```python
from build123d import *

# Parameters (mm, degrees)
CYLINDER_R        = 1.5
CYLINDER_DEPTH    = 8
CYLINDER002_R     = 1
CYLINDER002_DEPTH = 7
BOX005_W          = 11
BOX005_H          = 10
BOX005_DEPTH      = 6
FILLET001_R       = 3
BOX_W             = 14
BOX_H             = 30
BOX_DEPTH         = 24
BOX003_W          = 11
BOX003_H          = 3
BOX003_DEPTH      = 11
BOX004_W          = 11
BOX004_H          = 9
BOX004_DEPTH      = 7
CYLINDER001_R     = 1
CYLINDER001_DEPTH = 7
BOX002_W          = 11
BOX002_H          = 10
BOX002_DEPTH      = 11
BOX001_W          = 11
BOX001_H          = 51
BOX001_DEPTH      = 29
FILLET_R          = 10


with BuildPart() as side_cylinder:
    # Cylinder → Cylinder (new body)
    with BuildSketch(Plane(origin=(-1, -14.5, 12), x_dir=(0, 0, -1), z_dir=(1, 0, 0))):
        Circle(CYLINDER_R)
    extrude(amount=CYLINDER_DEPTH)


with BuildPart() as part_mirroring:
    # Part__Mirroring: instance of side cylinder
    add(side_cylinder.part.mirror(Plane(origin=(0, 0, 0), x_dir=(0, 1, 0), z_dir=(0, 0, 1))))


with BuildPart() as screw_hole_cylinder001:
    # Cylinder002 → Cylinder002 (new body)
    with BuildSketch(Plane(origin=(0, -18, 16), x_dir=(0, 0, -1), z_dir=(1, 0, 0))):
        Circle(CYLINDER002_R)
    extrude(amount=CYLINDER002_DEPTH)


with BuildPart() as cut001:
    # Box005 → Box005 (new body)
    with BuildSketch(Plane(origin=(-4, -23, 13), x_dir=(1, 0, 0), z_dir=(0, 0, 1))):
        with Locations((5.5, 5)):
            Rectangle(BOX005_W, BOX005_H)
    extrude(amount=BOX005_DEPTH)

    # Fillet001
    fillet001_edges = [cut001.edges().sort_by_distance(p)[0] for p in [
        (1.5, -23, 19),
        (1.5, -13, 19),
    ]]
    fillet(fillet001_edges, radius=FILLET001_R)

    # Cut001: cut screw hole cylinder001
    add(screw_hole_cylinder001.part, mode=Mode.SUBTRACT)


with BuildPart() as part_mirroring002:
    # Part__Mirroring002: instance of Cut001
    add(cut001.part.mirror(Plane(origin=(0, 0, 0), x_dir=(0, 1, 0), z_dir=(0, 0, 1))))


with BuildPart() as extract_cube:
    # Box → Box (new body)
    with BuildSketch(Plane(origin=(-1, -23, -12), x_dir=(1, 0, 0), z_dir=(0, 0, 1))):
        with Locations((7, 15)):
            Rectangle(BOX_W, BOX_H)
    extrude(amount=BOX_DEPTH)


with BuildPart() as pins_extraction_cube:
    # Box003 → Box003 (new body)
    with BuildSketch(Plane(origin=(-3, 0, -5.5), x_dir=(1, 0, 0), z_dir=(0, 0, 1))):
        with Locations((5.5, 1.5)):
            Rectangle(BOX003_W, BOX003_H)
    extrude(amount=BOX003_DEPTH)


with BuildPart() as wire_extract_cube:
    # Box004 → Box004 (new body)
    with BuildSketch(Plane(origin=(0, 17, -3.5), x_dir=(1, 0, 0), z_dir=(0, 0, 1))):
        with Locations((5.5, 4.5)):
            Rectangle(BOX004_W, BOX004_H)
    extrude(amount=BOX004_DEPTH)


with BuildPart() as screw_hole_cylinder:
    # Cylinder001 → Cylinder001 (new body)
    with BuildSketch(Plane(origin=(0, 15, 10), x_dir=(0, 0, -1), z_dir=(1, 0, 0))):
        Circle(CYLINDER001_R)
    extrude(amount=CYLINDER001_DEPTH)


with BuildPart() as part_mirroring001:
    # Part__Mirroring001: instance of screw hole cylinder
    add(screw_hole_cylinder.part.mirror(Plane(origin=(0, 0, 0), x_dir=(0, 1, 0), z_dir=(0, 0, 1))))


with BuildPart() as extract_fusion:
    # Box002 → Box002 (new body)
    with BuildSketch(Plane(origin=(0, 7, -5.5), x_dir=(1, 0, 0), z_dir=(0, 0, 1))):
        with Locations((5.5, 5)):
            Rectangle(BOX002_W, BOX002_H)
    extrude(amount=BOX002_DEPTH)

    # Fusion: union extract cube, pins extraction cube, wire extract cube, Part__Mirroring001, screw hole cylinder
    add(extract_cube.part)
    add(pins_extraction_cube.part)
    add(wire_extract_cube.part)
    add(part_mirroring001.part)
    add(screw_hole_cylinder.part)


with BuildPart() as body_fusion:
    # Box001 → Box001 (new body)
    with BuildSketch(Plane(origin=(-4, -23, -14.5), x_dir=(1, 0, 0), z_dir=(0, 0, 1))):
        with Locations((5.5, 25.5)):
            Rectangle(BOX001_W, BOX001_H)
    extrude(amount=BOX001_DEPTH)

    # Fillet
    fillet_edges = [body_fusion.edges().sort_by_distance(p)[0] for p in [
        (1.5, 28, -14.5),
        (1.5, 28, 14.5),
    ]]
    fillet(fillet_edges, radius=FILLET_R)

    # Cut: cut extract fusion
    add(extract_fusion.part, mode=Mode.SUBTRACT)

    # Fusion001: union Part__Mirroring, side cylinder, Part__Mirroring002, Cut001
    add(part_mirroring.part)
    add(side_cylinder.part)
    add(part_mirroring002.part)
    add(cut001.part)


solid = body_fusion.part
```
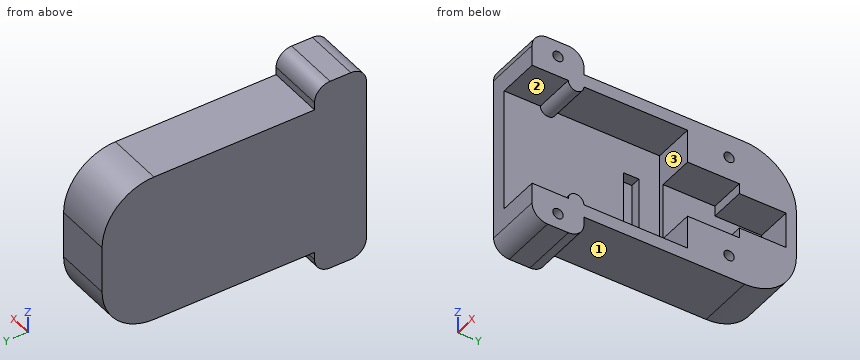
CAD build for the part. Positions are in the model's coordinates, mm. Face numbers are marked on the shaded views. A direction names the side the tool comes from. Coordinates: 2 decimals unless noted, no trailing zeros. Order: outer loops, then holes, each group sorted by start corner. A loop starts at its lowest first (then second) coordinate and runs counter-clockwise, first axis right, second up. Notation, with made-up numbers: M 71,-12 L 78,-12 A21 cw 78,15 Z; hole C 24.25,65.25 d6. An arc over 180 degrees is marked long. Answer as CSV lines item,"result".
1) Cut at B-B (z = -0.5). List the corners of the cut face in (x, y).
Verdict:
outline,"M -4,-23 L -1,-23 L -1,0 L -3,0 L -3,3 L -1,3 L -1,7 L 0,7 L 0,26 L 7,26 L 7,28 L -4,28 Z"
2) Cut at A-A (x = -1.75). List the corners of the cut face in (y, z).
Verdict:
outline,"M -23,-16 A3 ccw -20,-19 L -16,-19 A3 ccw -13,-16 L -13,-14.5 L 18,-14.5 A10 ccw 28,-4.5 L 28,4.5 A10 ccw 18,14.5 L -13,14.5 L -13,16 A3 ccw -16,19 L -20,19 A3 ccw -23,16 Z; hole M 0,-5.5 L 3,-5.5 L 3,5.5 L 0,5.5 Z"
3) Flat gauge pins, fed straight in: P1, Ø4, axis at x = 2, y = -3.5, coming from the -Z side; P2, Ø5.5, axis at x = 2, y = 3.5, coming from the +Z side; P3, Ø6, axis at y = -12.5, z = -7, coming from the +X side; P4, Ø1, axis at x = -2, z = 5, coming from the +Y side. Where does each tip first touch, or does it go through?
Verdict:
P1,"z = -14.5"
P2,"z = 14.5"
P3,"x = -1"
P4,"y = 28"
4) Cut at D-D (y = -9). List the corners of the cut face in (x, z).
Verdict:
outline,"M -4,-14.5 L 7,-14.5 L 7,-12 L -1,-12 L -1,12 L 7,12 L 7,14.5 L -4,14.5 Z"
5) Cut at C-C (x = 1.75). Give the number of separate pieces and of enclosed holes in the cut face, then the cut area to 3 significant figures.
Verdict:
separate pieces,"1"
enclosed holes,"4"
area,"620 mm2"
6) Drill centre lines: L1, parallel to Z at x = 6.5, y = 10.5; L2, parallel to Y at x = 3.25, z = 16; L3, parallel to Z at x = -0.25, y = -17.5. Where is each one in solid material? Low to high. Write a range as from..to.
Verdict:
L1,"-14.5..-5.5, 5.5..14.5"
L2,"-23..-19, -17..-13"
L3,"-19..-12, 12..19"
7) 3-axis set-ups, long thin cutter, end or side, ignore diameter. For the marked faces 1, 2 and 3: which of +Z, -Z, +X, -X, +Y, -Y reach the whole face in a straight line?
Verdict:
face 1,"-Z, +X, -X, +Y"
face 2,"+X, -Y"
face 3,"+X"
